Source: CAD feature listing. Evaluate the final solid. Frame: model axes, mm. Face numbers are marked on the shaded views. A direction names the side the tool comes from. Round coordinates to 2 decimals unless told otherwise and drop trailing zeros. Loops run counter-clockwise (first coordinate to the right, second up) from the corner with the lowest first, then second, coordinate; pieces in that order, holes last. Notation, with made-up numbers: (4.5, 74) -> (60.5, 74) arc R16 cw to (60.5, 100) -> close; hole circle Ø7 at (78.25, 78.25). An arc over 180 degrees is marked (long way). Put each result on its own line as item: value. Start each with the question number.
1. Cut plane C-C (x = -10.5). Return the cut outline in (y, z) (3 decimals), then the cut area to 3 significant figures.
2. Material intervals for L1, parallel to Y at x = 0, z = 7.5 (3 decimals); L2, parallel to Y at x = 2, z = 10 (3 decimals); L3, parallel to Y at x = -11, z = 2.5 (3 decimals), sorted ascending.
3. Cut plane A-A (y = 0). Return the cut outline in (x, z) (3 decimals).
4. Set-up query: the marked faces 4, 5 and 6. Return all of +Z, -Z, +X, -X, +Y, -Y with unobstructed straight access to the full face (end or side cutting, diameter ignored); none if empty.
5. Cut plane D-D (z = -14). Return the cut outline in (x, y) (3 decimals), then the cut area to 3 significant figures.
6. Cut plane B-B (x = 0). State how many separate pieces and enclosed holes the cut face has, then the cut area to 3 significant figures.
7. Draft query along X for the marked faces 1, 2 and 3. Return one class per face: pulls with the +X half, pulls with the -X half, needs draft (parallel to the pull), parting line crosses it, or undercut.
8. Contact query for flat-ended pins moving along their axis: pin 1 (15.5 mm diameter, centred on x = -5.5, y = 0, fed in from -Z); pin 2 (5 mm diameter, centred on x = 2, y = -13.5, fed in from +Z); pin 3 (8 mm diameter, centred on y = 7.5, z = 4.5, fed in from -X); pin 4 (15 mm diameter, centred on x = -1.5, z = -7.5, fed in from +Y). Output: stop coordinate, or through.
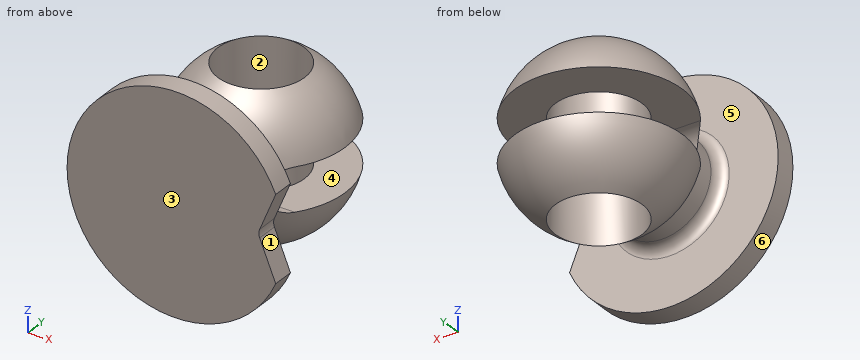
```python
from build123d import *

# Parameters (mm, degrees)
F1_R      = 6.35
F2_DEPTH  = 12.7
F5_R      = 15.875
F6_DEPTH  = 3.175
F8_R      = 7.1374
F9_DEPTH  = 7.9502
F13_DEPTH = 25.4
F15_R     = 1.5875
F17_DEPTH = 3.175


with BuildPart() as f2:
    # F1 (on Top) → F2 (new body, symmetric)
    with BuildSketch(Plane.XY):
        Circle(F1_R)
    extrude(amount=F2_DEPTH, both=True)


with BuildPart() as f3:
    # F0 (on Front) → F3 (revolve)
    with BuildSketch(Plane.XZ):
        with BuildLine():
            Line((0, 12.7), (0, -12.7))
            ThreePointArc((0, -12.7), (12.7, 0), (0, 12.7))
        make_face()
    revolve(axis=Axis((0, 0, 0), (0, 0, 1)))

    # F4: cut F2
    add(f2.part, mode=Mode.SUBTRACT)


with BuildPart() as f6:
    # F5 (on Front) → F6 (new body)
    with BuildSketch(Plane.XZ):
        Circle(F5_R)
    extrude(amount=F6_DEPTH)


with BuildPart() as f6_1:
    # F7: moved
    add(f6.part.moved(Location((0, -15.24, 0))))


with BuildPart() as f9:
    # F8 (on face) → F9 (new body)
    with BuildSketch(Plane.XZ.offset(18.415)):
        Circle(F8_R)
    extrude(amount=F9_DEPTH)


with BuildPart() as f9_1:
    # F10: moved
    add(f9.part.moved(Location((0, 7.9502, 0))))


with BuildPart() as f3_1:
    add(f3.part)

    # F11: union F6, F9
    add(f6_1.part)
    add(f9_1.part)


with BuildPart() as f13:
    # F12 (on Right) → F13 (new body, symmetric)
    with BuildSketch(Plane.YZ):
        with BuildLine():
            Line((27.5953571579, 3.175), (-7.3296428421, 3.175))
            ThreePointArc((-7.3296428421, 3.175), (-10.5046428421, 0), (-7.3296428421, -3.175))
            Line((-7.3296428421, -3.175), (27.5953571579, -3.175))
            Line((27.5953571579, -3.175), (27.5953571579, 3.175))
        make_face()
    extrude(amount=F13_DEPTH, both=True)


with BuildPart() as f3_2:
    add(f3_1.part)

    # F14: cut F13
    add(f13.part, mode=Mode.SUBTRACT)

    # F15
    f15_edges = [f3_2.edges().sort_by_distance(p)[0] for p in [
        (-7.1374, -15.24, 0),
    ]]
    fillet(f15_edges, radius=F15_R)


with BuildPart() as f17:
    # F16 (on face) → F17 (new body, symmetric)
    with BuildSketch(Plane.XZ.offset(18.415)):
        with BuildLine():
            Line((17.810190469, 14.0325875707), (12.2493412421, 0.6075099489))
            ThreePointArc((12.2493412421, 0.6075099489), (12.1285, 0), (12.2493412421, -0.6075099489))
            Line((12.2493412421, -0.6075099489), (17.810190469, -14.0325875707))
            Line((17.810190469, -14.0325875707), (17.810190469, 14.0325875707))
        make_face()
    extrude(amount=F17_DEPTH, both=True)


with BuildPart() as f3_3:
    add(f3_2.part)

    # F18: cut F17
    add(f17.part, mode=Mode.SUBTRACT)


solid = f3_3.part
```
Solution:
1. outline: (-18.415, -11.907) -> (-15.24, -11.907) -> (-15.24, 11.907) -> (-18.415, 11.907) -> close; (-6.4, -3.175) arc R7.144 ccw to (6.4, -3.175) -> close; (-6.4, 3.175) -> (6.4, 3.175) arc R7.144 ccw to start
1. area: 148 mm^2
2. L1: y = -18.415 to -14.662, -10.249 to -6.35, 6.35 to 10.249
2. L2: y = -18.415 to -15.24, -7.569 to -6.027, 6.027 to 7.569
2. L3: y = -18.415 to -15.24
3. outline: (-12.297, -3.175) arc R12.7 ccw to (-6.35, -10.999) -> (-6.35, -3.175) -> close; (-12.297, 3.175) -> (-6.35, 3.175) -> (-6.35, 10.999) arc R12.7 ccw to start; (6.35, -10.999) arc R12.7 ccw to (12.297, -3.175) -> (6.35, -3.175) -> close; (6.35, 3.175) -> (12.297, 3.175) arc R12.7 ccw to (6.35, 10.999) -> close
4. face 4: +X, -X, +Y
4. face 5: none
4. face 6: +Y, -Y
5. outline: (-7.484, -18.415) -> (7.484, -18.415) -> (7.484, -15.24) -> (-7.484, -15.24) -> close
5. area: 47.5 mm^2
6. separate pieces: 3
6. enclosed holes: 0
6. area: 285 mm^2
7. face 1: pulls with the +X half
7. face 2: undercut
7. face 3: needs draft
8. pin 1: stops at z = -11
8. pin 2: stops at z = 15.87
8. pin 3: stops at x = -11.72
8. pin 4: stops at y = 12.3
